Verification items for the finished model (mm, model axes). Face numbers are marked on the shaded views. A direction names the side the tool comes from. Round coordinates to 2 decimals unless told otherwise and drop trailing zeros. Order: outer loops, then holes, each group sorted by start corner. A loop starts at its lowest first (then second) coordinate and runs counter-clockwise, first axis right, second up. Notation, with made-up numbers: M 67,-14.75 L 71,-14.75 A34 ccw 71,19.25 Z; hole C 26.25,-13.5 d11. An arc over 180 degrees is marked long. Answer as a JSON object with one key per item and string values. Group by question number.
```python
from build123d import *

# Parameters (mm, degrees)
F0_W     = 16
F0_H     = 10
F1_DEPTH = 7.2
F2_W     = 5
F2_H     = 3
F3_DEPTH = 5
F4_R     = 1.3
F5_R     = 1.5
F6_DEPTH = 0.5


with BuildPart() as f1:
    # F0 (on Top) → F1 (new body)
    with BuildSketch(Plane.XY):
        Rectangle(F0_W, F0_H)
    extrude(amount=F1_DEPTH)

    # F2 (on face) → F3 (join)
    with BuildSketch(Plane.XY.offset(7.2)):
        with Locations((1.069713, 0)):
            Rectangle(F2_W, F2_H)
    extrude(amount=F3_DEPTH)

    # F4
    f4_edges = [f1.edges().sort_by_distance(p)[0] for p in [
        (-1.430287, 0, 12.2),
        (3.569713, 0, 12.2),
    ]]
    fillet(f4_edges, radius=F4_R)

    # F5 (on face) → F6 (join)
    with BuildSketch(Plane.XY.offset(7.2)):
        Polygon((0, 5), (-8, 5), (-12.830287, 4.792277), (-12.830287, 0), (-12.830287, -4.792277), (-8, -5), (0, -5), (8, -5), (12.830287, -4.792277), (12.830287, 0), (12.830287, 4.792277), (8, 5), align=None)
        with Locations((-10.3, 0)):
            Circle(F5_R, mode=Mode.SUBTRACT)
        with Locations((10.3, 0)):
            Circle(F5_R, mode=Mode.SUBTRACT)
    extrude(amount=-F6_DEPTH)


solid = f1.part
```
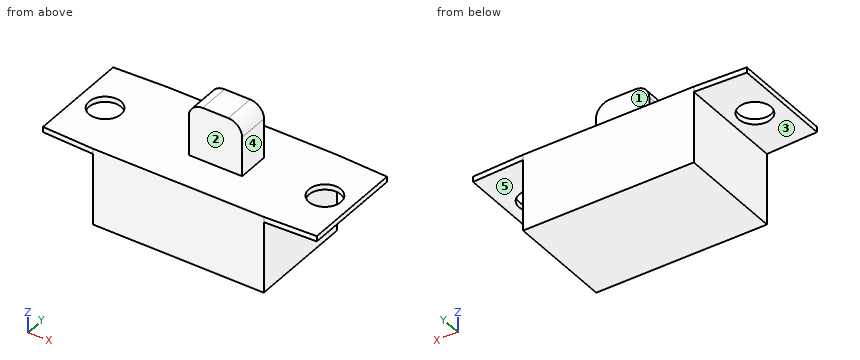
Q1. Cross-section at A-A, the plane x = 1. Record the cut outline in (y, z).
Q2. Gauge pin test, flat ends, axial feed: pin 1 Ø1 at (y, z) = (-1, 8.5) entering from +X; pin 2 Ø5 at (x, y) = (10.3, 0) entering from +Z; pin 3 Ø5.5 at (y, z) = (-0.5, 3) entering from +X. Record the tip position at first contact, or that the pin passes through.
Q3. Thickness scan on line 1 (X direction, y = 1.25, z = 3.5); line 2 (Z direction, x = 6.75, y = 0); line 3 (Z direction, x = -11.5, y = 4). Record the ranges inside material, lowest first. Write a range as from..to.
Q4. Cross-section at D-D, the plane y = 4. Record the cut outline in (x, z).
Q5. Tool access check on the marked faces 1, 2, 3, 4 and 5. Record the directions out of +Z, -Z, +X, -X, +Y, -Y that give a thin tool (end or side, any length) a straight path to the whole face; none if there is none.
Q6. Cross-section at C-C, the plane x = 9.5. Record the cut outline in (y, z), then the cut area to 3 significant figures.
Q7. Cross-section at B-B, the plane y = 0.5. Record the cut outline in (x, z).
Conclusion:
{
 "1": {"outline": "M -5,0 L 5,0 L 5,7.2 L 1.5,7.2 L 1.5,12.2 L -1.5,12.2 L -1.5,7.2 L -5,7.2 Z"},
 "2": {"pin 1": "x = 3.57", "pin 2": "z = 7.2", "pin 3": "x = 8"},
 "3": {"line 1": "-8..8", "line 2": "0..7.2", "line 3": "6.7..7.2"},
 "4": {"outline": "M -12.83,6.7 L -8,6.7 L -8,0 L 8,0 L 8,6.7 L 12.83,6.7 L 12.83,7.2 L -12.83,7.2 Z"},
 "5": {"face 1": "+Z, +X, -X, +Y", "face 2": "+Z, +X, -X, -Y", "face 3": "-Z, -X, +Y, -Y", "face 4": "+Z, +X, +Y, -Y", "face 5": "-Z, +X, +Y, -Y"},
 "6": {"outline": "M -4.94,6.7 L -1.27,6.7 L -1.27,7.2 L -4.94,7.2 Z; M 1.27,6.7 L 4.94,6.7 L 4.94,7.2 L 1.27,7.2 Z", "area": "3.67 mm2"},
 "7": {"outline": "M -12.83,6.7 L -11.71,6.7 L -11.71,7.2 L -12.83,7.2 Z; M -8.89,6.7 L -8,6.7 L -8,0 L 8,0 L 8,6.7 L 8.89,6.7 L 8.89,7.2 L 3.57,7.2 L 3.57,10.9 A1.3 ccw 2.27,12.2 L -0.13,12.2 A1.3 ccw -1.43,10.9 L -1.43,7.2 L -8.89,7.2 Z; M 11.71,6.7 L 12.83,6.7 L 12.83,7.2 L 11.71,7.2 Z"}
}
